Autodesk Inventor part; units mm, degrees
ref_plane "YZ Plane" through (0, 0, 0) normal (1, 0, 0) x (0, 1, 0)
ref_plane "XZ Plane" through (0, 0, 0) normal (0, 1, 0) x (-1, 0, 0)
ref_plane "XY Plane" through (0, 0, 0) normal (0, 0, 1) x (1, 0, 0)
sketch "Szkic1" plane through (0, 0, 0) normal (0, 1, 0) x (-1, 0, 0)
  line L0 (-35, -68) -> (35, -68)
  line L1 (35, -68) -> (35, 68)
  line L2 (35, 68) -> (-35, 68)
  line L3 (-35, 68) -> (-35, -68)
  line L4 (-35, -68) -> (35, 68) construction
  line L5 (35, -68) -> (-35, 68) construction
  point P0 (0, 0)
  dimension "d0" = 70
  dimension "d1" = 136
extrude "Wyciągnięcie proste1" add sketch "Szkic1" along normal blind 2.5
sketch "Szkic2" plane through (0, 2.5, 0) normal (0, 1, 0) x (1, 0, 0)
  line L0 (-52.8, 0) -> (71.8, 0)
  line L1 (35, -68) -> (35, 68)
  line L2 (55, -35) -> (35, -35)
  line L3 (35, -35) -> (35, 35)
  line L4 (35, 35) -> (55, 35)
  line L5 (55, 35) -> (55, -35)
  line L6 (55, -35) -> (35, 35) construction
  line L7 (35, -35) -> (55, 35) construction
  point P0 (0, 0)
  point P1 (45, 0)
  dimension "d4" = 20
  dimension "d5" = 70
extrude "Wyciągnięcie proste2" add sketch "Szkic2" against normal up to surface (2.5 mm away)
sketch "Szkic3" plane through (0, 2.5, 0) normal (0, 1, 0) x (1, 0, 0)
  circle A0 centre (-25, 64) radius 1.3
  line L0 (35, 68) -> (-35, 68)
  line L1 (-35, -68) -> (35, -68)
  line L2 (-35, 68) -> (-35, -68)
  circle A1 centre (14.5, 64) radius 1.3
  circle A2 centre (-25, -64) radius 1.3
  circle A3 centre (14.5, -64) radius 1.3
  point P0 (0, 0)
  dimension "d8" = 2.6
  dimension "d9" = 4
  dimension "d10" = 136
  dimension "d13" = 39.5
  dimension "d16" = 128
  dimension "d19" = 10
extrude "Wyciągnięcie proste3" cut sketch "Szkic3" against normal up to next
sketch "Szkic4" plane through (0, 2.5, 0) normal (0, 1, 0) x (1, 0, 0)
  line L0 (-23, -65) -> (12, -65)
  line L1 (12, -65) -> (12, -62.5)
  line L2 (12, -62.5) -> (-23, -62.5)
  line L3 (-23, -62.5) -> (-23, -65)
  line L4 (-23, -65) -> (12, -62.5) construction
  line L5 (12, -65) -> (-23, -62.5) construction
  line L6 (-35, -68) -> (35, -68)
  line L7 (-35, 68) -> (-35, -68)
  point P0 (0, 0)
  point P1 (-5.5, -63.75)
  dimension "d22" = 35
  dimension "d23" = 2.5
  dimension "d24" = 3
  dimension "d25" = 12
extrude "Wyciągnięcie proste4" add sketch "Szkic4" along normal blind 9
sketch "Szkic5" plane through (0, 2.5, 0) normal (0, 1, 0) x (1, 0, 0)
  line L0 (-29.5, -54) -> (-23.5, -54)
  line L1 (-23.5, -54) -> (-23.5, 27)
  line L2 (-23.5, 27) -> (-29.5, 27)
  line L3 (-29.5, 27) -> (-29.5, -54)
  line L4 (-29.5, -54) -> (-23.5, 27) construction
  line L5 (-23.5, -54) -> (-29.5, 27) construction
  line L6 (-35, -68) -> (35, -68)
  line L7 (-35, 68) -> (-35, -68)
  line L8 (17, -54) -> (23, -54)
  line L9 (23, -54) -> (23, 27)
  line L10 (23, 27) -> (17, 27)
  line L11 (17, 27) -> (17, -54)
  line L12 (17, -54) -> (23, 27) construction
  line L13 (23, -54) -> (17, 27) construction
  line L14 (35, -68) -> (35, -35)
  point P0 (0, 0)
  point P1 (-26.5, -13.5)
  point P2 (20, -13.5)
  dimension "d28" = 6
  dimension "d29" = 81
  dimension "d30" = 14
  dimension "d31" = 5.5
  dimension "d32" = 6
  dimension "d33" = 81
  dimension "d34" = 14
  dimension "d35" = 12
extrude "Wyciągnięcie proste5" add sketch "Szkic5" along normal blind 9
sketch "Szkic6" plane through (0, 2.5, 0) normal (0, 1, 0) x (1, 0, 0)
  line L0 (32.5, 55) -> (17.5, 55)
  line L1 (17.5, 55) -> (17.5, 62.5)
  line L2 (17.5, 62.5) -> (32.5, 62.5)
  line L3 (32.5, 62.5) -> (32.5, 55)
  line L4 (32.5, 55) -> (17.5, 62.5) construction
  line L5 (17.5, 55) -> (32.5, 62.5) construction
  line L6 (11, 62.5) -> (1, 62.5)
  line L7 (1, 62.5) -> (1, 55)
  line L8 (1, 55) -> (11, 55)
  line L9 (11, 55) -> (11, 62.5)
  line L10 (11, 62.5) -> (1, 55) construction
  line L11 (1, 62.5) -> (11, 55) construction
  line L12 (35, 35) -> (35, 68)
  line L13 (35, 68) -> (-35, 68)
  point P0 (0, 0)
  point P1 (25, 58.75)
  point P2 (6, 58.75)
  dimension "d38" = 15
  dimension "d39" = 7.5
  dimension "d40" = 10
  dimension "d41" = 7.5
  dimension "d42" = 6.5
  dimension "d43" = 2.5
  dimension "d44" = 5.5
  dimension "d45" = 5.5
extrude "Wyciągnięcie proste6" add sketch "Szkic6" along normal blind 11
sketch "Szkic7" plane through (0, 2.5, 0) normal (0, 1, 0) x (1, 0, 0)
  line L0 (-0.5, 65.5) -> (-14.5, 65.5)
  line L1 (-14.5, 65.5) -> (-14.5, 63)
  line L2 (-14.5, 63) -> (-0.5, 63)
  line L3 (-0.5, 63) -> (-0.5, 65.5)
  line L4 (-0.5, 65.5) -> (-14.5, 63) construction
  line L5 (-14.5, 65.5) -> (-0.5, 63) construction
  line L6 (35, 68) -> (-35, 68)
  line L7 (-35, 68) -> (-35, -68)
  point P0 (0, 0)
  point P1 (-7.5, 64.25)
  dimension "d48" = 14
  dimension "d49" = 2.5
  dimension "d50" = 2.5
  dimension "d51" = 20.5
extrude "Wyciągnięcie proste7" add sketch "Szkic7" along normal blind 9
sketch "Szkic8" plane through (0, 0, 0) normal (0, -1, 0) x (1, 0, 0)
  line L0 (20, 56) -> (-23, 56)
  line L1 (-23, 56) -> (-23, -30)
  line L2 (-23, -30) -> (20, -30)
  line L3 (20, -30) -> (20, 56)
  line L4 (20, 56) -> (-23, -30) construction
  line L5 (-23, 56) -> (20, -30) construction
  line L6 (-35, 68) -> (35, 68)
  line L7 (-35, -68) -> (-35, 68)
  point P0 (0, 0)
  point P1 (-1.5, 13)
  dimension "d54" = 43
  dimension "d55" = 86
  dimension "d56" = 12
  dimension "d57" = 12
extrude "Wyciągnięcie proste8" add sketch "Szkic8" along normal blind 18
equation "\"d16\" = d10 - 2 * d9"
equation "\"d45\" = d44"
properties part number "pcb"
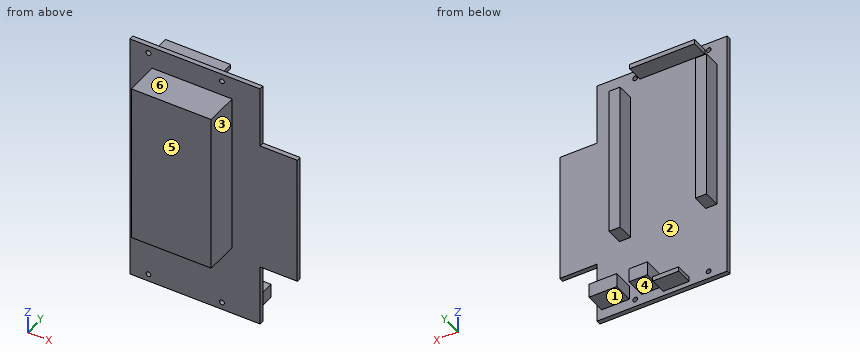
Part model, mm, in its own coordinate system. Face numbers are marked on the shaded views. A direction names the side the tool comes from. Round coordinates to 2 decimals unless told otherwise and drop trailing zeros. Order: outer loops, then holes, each group sorted by start corner. A loop starts at its lowest first (then second) coordinate and runs counter-clockwise, first axis right, second up. Notation, with made-up numbers: M 33,85 L 62,85 A35 cw 62,123 Z; hole C 64,-28 d2. An arc over 180 degrees is marked long. Put each result on its own line as item: value. Start each with the question number.
1. Tool access for the marked faces 4, 5 and 6: list every direction of +Z, -Z, +X, -X, +Y, -Y with a clear straight run to the whole face (end or side of a thin tool).
2. Slice it at B-B on x = -19. List the corners of the cut face in (y, z), then the cut area to 3 significant figures.
3. Slice it at D-D on y = -8. List the corners of the cut face in (x, z), then the cut area to 3 significant figures.
4. Slice it at A-A on y = 9.5. List the corners of the cut face in (x, z), then the cut area to 3 significant figures.
5. Drill centre lines: probe 1 along X at (y, z) = (0.9, 64); probe 2 along Z at (x, y) = (-25, 1.6); probe 3 along Z at (x, y) = (4.5, 8). Where is each one in solid material? Low to high. Write a range as [from, to].
6. Drop flat-ended pins along their axis: pin 1 (2.5 mm diameter, centred on x = -6.5, y = 8.5, fed in from +Z); pin 2 (14.5 mm diameter, centred on x = 1.5, y = -12, fed in from -Z); pin 3 (8 mm diameter, centred on y = 7, z = -57.5, fed in from +X). Give the stop position or say it passes through.
7. Slice it at C-C on z = 38. List the corners of the cut face in (x, y).
8. Two-plate mould, pull along X, no slides. Class the marked faces 1, 2 and 3: +X half, -X half, draft (parallel to the pull), parting line (faces both ways), or undercut.
Findings:
1. face 4: -Z, +X, -X, +Y
1. face 5: +Z, -Z, +X, -X, -Y
1. face 6: +Z, +X, -X, -Y
2. outline: M -18,-30 L 0,-30 L 0,-68 L 2.5,-68 L 2.5,62.5 L 11.5,62.5 L 11.5,65 L 2.5,65 L 2.5,68 L 0,68 L 0,56 L -18,56 Z
2. area: 1,910 mm2
3. outline: M -23,-30 L 20,-30 L 20,56 L -23,56 Z
3. area: 3,700 mm2
4. outline: M -29.5,-27 L -23.5,-27 L -23.5,54 L -29.5,54 Z; M -23,62.5 L 12,62.5 L 12,65 L -23,65 Z; M -14.5,-65.5 L -0.5,-65.5 L -0.5,-63 L -14.5,-63 Z; M 1,-62.5 L 11,-62.5 L 11,-55 L 1,-55 Z; M 17,-27 L 23,-27 L 23,54 L 17,54 Z; M 17.5,-62.5 L 32.5,-62.5 L 32.5,-55 L 17.5,-55 Z
4. area: 1,280 mm2
5. probe 1: [-35, -26.3], [-23.7, 13.2], [15.8, 35]
5. probe 2: [-68, -65.3], [-62.7, 62.7], [65.3, 68]
5. probe 3: [-62.5, -55], [62.5, 65]
6. pin 1: z = 65
6. pin 2: z = -30
6. pin 3: x = 32.5
7. outline: M -35,0 L -23,0 L -23,-18 L 20,-18 L 20,0 L 35,0 L 35,2.5 L 23,2.5 L 23,11.5 L 17,11.5 L 17,2.5 L -23.5,2.5 L -23.5,11.5 L -29.5,11.5 L -29.5,2.5 L -35,2.5 Z
8. face 1: draft
8. face 2: undercut
8. face 3: +X half
